Geometry check sheet. Reference: the model listing, model coordinates, mm. Face numbers are marked on the shaded views. A direction names the side the tool comes from. Round coordinates to 2 decimals unless told otherwise and drop trailing zeros. Write each loop counter-clockwise with the first axis right and the second up, starting at its lowest first coordinate (ties: lowest second). Pieces come first, ordered by that corner, then holes. Notation, with made-up numbers: (11, -27.5) -> (51, -27.5) arc R17 ccw to (51, -2.5) -> close; hole circle Ø11 at (52, 60.5). An arc over 180 degrees is marked (long way). One line per question, with ' | ' between items.
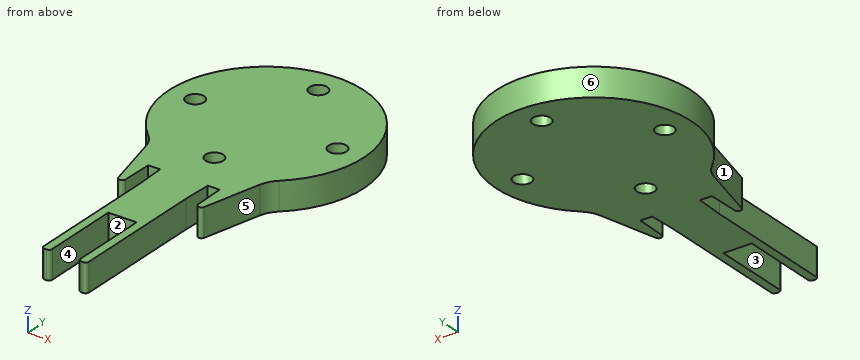
Autodesk Inventor part; units mm, degrees
ref_plane "YZ Plane" through (0, 0, 0) normal (1, 0, 0) x (0, 1, 0)
ref_plane "XZ Plane" through (0, 0, 0) normal (0, 1, 0) x (-1, 0, 0)
ref_plane "XY Plane" through (0, 0, 0) normal (0, 0, 1) x (1, 0, 0)
ref_plane "Work Plane1" through (0, -7.809, 0) normal (-1, 0, 0) x (0, 0, 1)
ref_plane "Work Plane2" through (0, 0, 1.5875) normal (0, 0, 1) x (1, 0, 0)
sketch "Sketch1" plane through (0, 0, 0) normal (0, 0, 1) x (1, 0, 0)
  line L0 (-2.54, -8.19) -> (2.54, -8.19)
  line L1 (2.54, -8.19) -> (2.54, 8.19)
  line L2 (-2.54, 8.19) -> (-2.54, -8.19)
  line L3 (-2.54, -8.19) -> (2.54, 8.19) construction
  line L4 (2.54, -8.19) -> (-2.54, 8.19) construction
  circle A0 centre (0, 16.6545) radius 2.5 construction
  circle A1 centre (0, 16.6545) radius 5
  arc A2 (6.8029, 15.0051) -> (-6.8044, 15.0114) centre (0, 16.6545) ccw
  line L5 (-2.54, 8.19) -> (-2.54, 10.2591)
  line L6 (2.54, 8.19) -> (2.54, 10.2869)
  line L7 (0, 0) -> (0, 10.7842) construction
  line L8 (-2.54, 10.2591) -> (-3.9944, 10.2511)
  line L9 (2.54, 10.2869) -> (3.9944, 10.2948)
  line L10 (-3.9944, 10.2511) -> (-4.1214, 3.9003)
  line L11 (3.9944, 10.2948) -> (4.1214, 3.9454)
  line L12 (-4.1214, 3.9003) -> (-6.8044, 15.0114)
  line L13 (4.1214, 3.9454) -> (6.8029, 15.0051)
  line L14 (0, 0) -> (0, 22.9511) construction
  point P0 (-3.2672, 10.2551)
  dimension "d16" = 0
  dimension "d2" = 5
  dimension "d3" = 10
  dimension "d4" = 14
  dimension "d8" = 1.5815
  dimension "d9" = 1.5815
  dimension "d10" = 6.35
  dimension "d11" = 6.35
  dimension "d18" = 1.4545
  dimension "d19" = 1.4545
  dimension "d31" = 2.54
  dimension "d32" = 2.54
  dimension "d33" = 0
extrude "Plate1" add sketch "Sketch1" along normal blind 3.175
sketch "Sketch2" plane through (0, 0, 0) normal (0, 0, -1) x (-1, 0, 0)
  circle A0 centre (0, 16.6545) radius 5
  line L0 (-3.9944, 10.2948) -> (-4.1214, 3.9454)
  line L1 (-2.54, 10.2869) -> (-3.9944, 10.2948)
  line L2 (-2.54, -8.19) -> (-2.54, 10.2869)
  line L3 (2.54, -8.19) -> (-2.54, -8.19)
  line L4 (2.54, 10.2591) -> (2.54, -8.19)
  line L5 (3.9944, 10.2511) -> (2.54, 10.2591)
  line L6 (4.1214, 3.9003) -> (3.9944, 10.2511)
  line L7 (6.8044, 15.0114) -> (4.1214, 3.9003)
  arc A1 (6.8044, 15.0114) -> (-6.8029, 15.0051) centre (0, 16.6545) ccw
  line L8 (-4.1214, 3.9454) -> (-6.8029, 15.0051)
  line L9 (-1.5875, -17.19) -> (1.5875, -17.19)
  line L10 (1.5875, -17.19) -> (1.5875, 0.81)
  line L11 (1.5875, 0.81) -> (-1.5875, 0.81)
  line L12 (-1.5875, 0.81) -> (-1.5875, -17.19)
  line L13 (-1.5875, -17.19) -> (1.5875, 0.81) construction
  line L14 (1.5875, -17.19) -> (-1.5875, 0.81) construction
  point P0 (0, 0)
  point P1 (0, -8.19)
  dimension "d14" = 3.175
extrude "Extrusion1" cut sketch "Sketch2" against normal blind 25.4 contours L12 L11 L10 L3 | L3 L10 L9 L12
sketch "Sketch3" plane through (0, 0, 3.175) normal (0, 0, 1) x (1, 0, 0)
  circle A0 centre (-37.757, 0) radius 3
  line L0 (-39.3445, -2.5456) -> (-36.1695, -2.5456)
  line L1 (-36.1695, -2.5456) -> (-36.1695, 2.5456)
  line L2 (-36.1695, 2.5456) -> (-39.3445, 2.5456)
  line L3 (-39.3445, 2.5456) -> (-39.3445, -2.5456)
  line L4 (-39.3445, -2.5456) -> (-36.1695, 2.5456) construction
  line L5 (-36.1695, -2.5456) -> (-39.3445, 2.5456) construction
  circle A1 centre (-37.757, 0) radius 4
  point P0 (0, 0)
  point P1 (-37.757, 3)
  point P2 (-37.757, 4)
  dimension "d35" = 8
  dimension "d28" = 6
  dimension "d29" = 3.175
  dimension "d30" = 5.0911
  dimension "d34" = 0.4545
  dimension "d36" = 1.4545
fillet "Fillet4" radius 0.381 6 edges at (-4.1214, 3.9003, 1.5875) (4.1214, 3.9454, 1.5875) (-2.54, -8.19, 1.5875) (-1.5875, -8.19, 1.5875) (1.5875, -8.19, 1.5875) (2.54, -8.19, 1.5875)
sketch "Sketch4" plane through (0, 0, 3.175) normal (0, 0, 1) x (1, 0, 0)
  arc A0 (2.159, -8.19) -> (2.54, -7.809) centre (2.159, -7.809) ccw
  line L0 (2.54, 10.2869) -> (2.54, -7.809)
  line L1 (3.9944, 10.2948) -> (2.54, 10.2869)
  line L2 (4.0627, 6.8835) -> (3.9944, 10.2948)
  arc A1 (4.0627, 6.8835) -> (4.8139, 6.8013) centre (4.4436, 6.8911) ccw
  line L3 (6.8029, 15.0051) -> (4.8139, 6.8013)
  arc A2 (6.8029, 15.0051) -> (-6.8044, 15.0114) centre (0, 16.6545) ccw
  line L4 (-4.8137, 6.7674) -> (-6.8044, 15.0114)
  arc A3 (-4.8137, 6.7674) -> (-4.0625, 6.8492) centre (-4.4434, 6.8568) ccw
  line L5 (-3.9944, 10.2511) -> (-4.0625, 6.8492)
  line L6 (-2.54, 10.2591) -> (-3.9944, 10.2511)
  line L7 (-2.54, -7.809) -> (-2.54, 10.2591)
  arc A4 (-2.54, -7.809) -> (-2.159, -8.19) centre (-2.159, -7.809) ccw
  line L8 (-1.9685, -8.19) -> (-2.159, -8.19)
  arc A5 (-1.9685, -8.19) -> (-1.5875, -7.809) centre (-1.9685, -7.809) ccw
  line L9 (-1.5875, -7.809) -> (-1.5875, 0.81)
  line L10 (-1.5875, 0.81) -> (1.5875, 0.81)
  line L11 (1.5875, 0.81) -> (1.5875, -7.809)
  arc A6 (1.5875, -7.809) -> (1.9685, -8.19) centre (1.9685, -7.809) ccw
  line L12 (2.159, -8.19) -> (1.9685, -8.19)
  circle A7 centre (0, 16.6545) radius 5
  point P0 (0, 0)
extrude "Extrusion2" add sketch "Sketch4" against normal up to surface (3.175 mm away) contours A7
sketch "Sketch5" plane through (0, 0, 3.175) normal (0, 0, 1) x (1, 0, 0)
  arc A0 (2.159, -8.19) -> (2.54, -7.809) centre (2.159, -7.809) ccw
  line L0 (2.54, 10.2869) -> (2.54, -7.809)
  line L1 (3.9944, 10.2948) -> (2.54, 10.2869)
  line L2 (4.0627, 6.8835) -> (3.9944, 10.2948)
  arc A1 (4.0627, 6.8835) -> (4.8139, 6.8013) centre (4.4436, 6.8911) ccw
  line L3 (6.8029, 15.0051) -> (4.8139, 6.8013)
  arc A2 (6.8029, 15.0051) -> (-6.8044, 15.0114) centre (0, 16.6545) ccw
  line L4 (-4.8137, 6.7674) -> (-6.8044, 15.0114)
  arc A3 (-4.8137, 6.7674) -> (-4.0625, 6.8492) centre (-4.4434, 6.8568) ccw
  line L5 (-3.9944, 10.2511) -> (-4.0625, 6.8492)
  line L6 (-2.54, 10.2591) -> (-3.9944, 10.2511)
  line L7 (-2.54, -7.809) -> (-2.54, 10.2591)
  arc A4 (-2.54, -7.809) -> (-2.159, -8.19) centre (-2.159, -7.809) ccw
  line L8 (-1.9685, -8.19) -> (-2.159, -8.19)
  arc A5 (-1.9685, -8.19) -> (-1.5875, -7.809) centre (-1.9685, -7.809) ccw
  line L9 (-1.5875, -7.809) -> (-1.5875, 0.81)
  line L10 (-1.5875, 0.81) -> (1.5875, 0.81)
  line L11 (1.5875, 0.81) -> (1.5875, -7.809)
  arc A6 (1.5875, -7.809) -> (1.9685, -8.19) centre (1.9685, -7.809) ccw
  line L12 (2.159, -8.19) -> (1.9685, -8.19)
  arc A7 (1.5644, 14.7045) -> (-1.5644, 14.7045) centre (0, 16.6545) ccw
  line L13 (1.5644, 14.7045) -> (-1.5644, 14.7045)
  point P0 (0, 0)
  point P1 (0, 19.1545)
  dimension "d40" = 5
  dimension "d44" = 4.45
extrude "Extrusion3" cut sketch "Sketch5" against normal blind 25.4 contours L13 A7
sketch "Sketch6" plane through (0, 0, 3.175) normal (0, 0, 1) x (1, 0, 0)
  circle A0 centre (-0.0066, 22.9731) radius 10.9474
  line L0 (3.9944, 10.2948) -> (2.54, 10.2869)
  point P0 (0, 0)
  dimension "d45" = 21.8948
  dimension "d46" = 12.7
extrude "Extrusion4" add sketch "Sketch6" against normal up to surface (3.175 mm away)
fillet "Fillet5" radius 3.175 2 edges at (-6.6204, 14.2495, 1.5875) (6.6225, 14.2611, 1.5875)
chamfer "Chamfer3" distance 0.127 distance2 3.175 1 edges at (-2.54, 10.2591, 1.5875) measured on face at (-3.5096, 10.2538, 1.0583)
chamfer "Chamfer4" distance 3.175 distance2 0.127 1 edges at (2.54, 10.2869, 1.5875) measured on face at (2.54, -1.7771, 1.0583)
sketch "Sketch7" plane through (0, 0, 3.175) normal (0, 0, 1) x (1, 0, 0)
  line L0 (-4.8137, 6.7674) -> (-6.3734, 13.2264)
  arc A0 (-4.8137, 6.7674) -> (-4.0625, 6.8492) centre (-4.4434, 6.8568) ccw
  line L1 (-3.9944, 10.2511) -> (-4.0625, 6.8492)
  line L2 (-2.667, 10.2584) -> (-3.9944, 10.2511)
  line L3 (-2.54, 7.0841) -> (-2.667, 10.2584)
  line L4 (-2.54, -7.809) -> (-2.54, 7.0841)
  arc A1 (-2.54, -7.809) -> (-2.159, -8.19) centre (-2.159, -7.809) ccw
  line L5 (-1.9685, -8.19) -> (-2.159, -8.19)
  arc A2 (-1.9685, -8.19) -> (-1.5875, -7.809) centre (-1.9685, -7.809) ccw
  line L6 (-1.5875, -7.809) -> (-1.5875, 0.81)
  line L7 (-1.5875, 0.81) -> (1.5875, 0.81)
  line L8 (1.5875, 0.81) -> (1.5875, -7.809)
  arc A3 (1.5875, -7.809) -> (1.9685, -8.19) centre (1.9685, -7.809) ccw
  line L9 (2.159, -8.19) -> (1.9685, -8.19)
  arc A4 (2.159, -8.19) -> (2.54, -7.809) centre (2.159, -7.809) ccw
  line L10 (2.54, 7.1119) -> (2.54, -7.809)
  line L11 (2.667, 10.2876) -> (2.54, 7.1119)
  line L12 (3.9944, 10.2948) -> (2.667, 10.2876)
  line L13 (4.0627, 6.8835) -> (3.9944, 10.2948)
  arc A5 (4.0627, 6.8835) -> (4.8139, 6.8013) centre (4.4436, 6.8911) ccw
  line L14 (6.3756, 13.2425) -> (4.8139, 6.8013)
  arc A6 (7.3326, 14.8503) -> (6.3756, 13.2425) centre (9.4612, 12.4944) ccw
  arc A7 (7.3326, 14.8503) -> (-7.3345, 14.84) centre (-0.0066, 22.9731) ccw
  arc A8 (-6.3734, 13.2264) -> (-7.3345, 14.84) centre (-9.4597, 12.4812) ccw
  circle A9 centre (-0.0066, 22.9731) radius 8
  point P0 (0, 0)
  point P1 (-0.0066, 14.9731)
  point P2 (-0.0066, 30.9731)
  point P3 (-8.0066, 22.9731)
  point P4 (7.9934, 22.9731)
  dimension "d56" = 16
hole "Hole1" at (-0.0066, 14.9731, 3.175) at (-0.0066, 30.9731, 3.175) at (-8.0066, 22.9731, 3.175) at (7.9934, 22.9731, 3.175) direction (0, 0, -1) diameter 2 end through all
equation "\"d18\" = d36"
equation "\"d19\" = d36"
equation "\"d62\" = Thickness"
equation "\"BendRadius\" = Thickness"
equation "\"BendReliefWidth\" = Thickness"
equation "\"BendReliefDepth\" = 0.5 * Thickness"
equation "\"CornerReliefSize\" = 4 * Thickness"
equation "\"MinimumRemnant\" = 2 * Thickness"
equation "\"TransitionRadius\" = BendRadius"
equation "\"JacobiRadiusSize\" = BendRadius"
equation "\"GapSize\" = Thickness"
equation "\"d12\" = BendRadius"
properties part number "8mm OD 6mm ID Rod End125Dynamixel"
(1) Sectioned sample at B-B on z = 0.8. Count the separate pieces of the cut face and the enclosed holes in it, then the cut area to 3 significant figures.
Resolved:
separate pieces: 1 | enclosed holes: 4 | area: 467 mm2
(2) Access from +Z, -Z, +X, -X, +Y, -Y to the whole of each face (thin tool, end or side, straight path). Record for the marked faces 1 and 2.
Resolved:
face 1: +Z, -Z, -X, -Y | face 2: +Z, -Z, -Y
(3) Sectioned sample at A-A on y = -3. Record the cut outline in (x, z) (1 decimal).
Resolved:
outline: (-2.5, 0) -> (-1.6, 0) -> (-1.6, 3.2) -> (-2.5, 3.2) -> close; (1.6, 0) -> (2.5, 0) -> (2.5, 3.2) -> (1.6, 3.2) -> close
(4) Draft check along X on the marked faces 3, 4, 5 and 6. Enter one of: +X half, -X half, draft (parallel to the pull), parting line (faces both ways), or undercut.
Resolved:
face 3: undercut | face 4: undercut | face 5: +X half | face 6: parting line
(5) Sectioned sample at D-D on y = 25.5. Record the cut outline in (x, z) (3 decimals), then the cut area to 3 significant figures.
Resolved:
outline: (-10.658, 0) -> (10.645, 0) -> (10.645, 3.175) -> (-10.658, 3.175) -> close | area: 67.6 mm2
(6) Sectioned sample at C-C on x = 8.5. Record the cut outline in (y, z) (3 decimals).
Resolved:
outline: (16.082, 0) -> (22.111, 0) -> (22.111, 3.175) -> (16.082, 3.175) -> close; (23.835, 0) -> (29.864, 0) -> (29.864, 3.175) -> (23.835, 3.175) -> close
(7) Go/stop test with flat-tipped pins: pin 1 (1.8 mm diameter, centred on x = -8.01, y = 22.97, fed in from +Z); pin 2 (1 mm diameter, centred on y = -3.5, z = 2, fed in from -X); pin 3 (1 mm diameter, centred on x = 8.5, z = 1, fed in from -Y); pin 4 (1 mm diameter, centred on y = -1.5, z = 1.5, fed in from +X). Record where each tip stops, or that it passes through.
Resolved:
pin 1: passes through | pin 2: stops at x = -2.54 | pin 3: stops at y = 15.51 | pin 4: stops at x = 2.54
(8) Material ranges on line 1 (X direction, y = 7, z = 0.95); line 2 (X direction, y = 10, z = 1.2); line 3 (X direction, y = -5, z = 2.8), recorded low to high.
Resolved:
line 1: x = -4.87 to -4.06, -2.54 to 2.54, 4.06 to 4.86 | line 2: x = -5.59 to -4, -2.66 to 2.66, 4 to 5.59 | line 3: x = -2.54 to -1.59, 1.59 to 2.54
